CAD build for the part. Positions are in the model's coordinates, mm. Give positions to 0.01 mm unless a question says otherwise; leave off trailing zeros. Write each loop counter-clockwise with the first axis right and the second up, starting at its lowest first coordinate (ties: lowest second). Pieces come first, ordered by that corner, then holes. Notation, with made-up numbers: (-9.75, 60) - (44.25, 60) arc R18 ccw to (44.25, 75) - close; hole circle Ø6 at (3, 1.25). An arc over 180 degrees is marked (long way). Answer as a JSON object with one key per item and string values.
Autodesk Inventor part; units mm, degrees
ref_plane "YZ Plane" through (0, 0, 0) normal (1, 0, 0) x (0, 1, 0)
ref_plane "XZ Plane" through (0, 0, 0) normal (0, 1, 0) x (-1, 0, 0)
ref_plane "XY Plane" through (0, 0, 0) normal (0, 0, 1) x (1, 0, 0)
sketch "Esquisse1" plane through (0, 0, 0) normal (0, 1, 0) x (-1, 0, 0)
  line L0 (100, 500) -> (-100, 500)
  line L1 (-100, 500) -> (-100, -500)
  line L2 (-100, -500) -> (100, -500)
  line L3 (100, -500) -> (100, 500)
  point P0 (0, 0)
  dimension "d0" = 1000
  dimension "d1" = 200
  dimension "d4" = 500
  dimension "d5" = 100
extrude "Extrusion1" add sketch "Esquisse1" along normal blind 10
sketch "Esquisse2" plane through (0, 10, 0) normal (0, 1, 0) x (1, 0, 0)
  line L0 (100, -500) -> (100, 500)
  line L1 (100, -340) -> (40, -300)
  line L2 (40, -300) -> (40, 300)
  line L3 (40, 300) -> (100, 340)
  line L4 (-100, 500) -> (-100, -500)
  point P0 (0, 0)
  dimension "d6" = 600
  dimension "d7" = 300
  dimension "d8" = 140
  dimension "d9" = 160
  dimension "d10" = 160
extrude "Extrusion2" cut sketch "Esquisse2" against normal through all
fillet "Congé1" radius 20 4 edges at (40, 5, 300) (100, 5, 340) (40, 5, -300) (100, 5, -340)
sketch "Esquisse3" plane through (0, 10, 0) normal (0, 1, 0) x (1, 0, 0)
  circle A0 centre (-60, -485) radius 1.5
  circle A1 centre (60, -485) radius 1.5
  circle A2 centre (-60, 485) radius 1.5
  circle A3 centre (60, 485) radius 1.5
  line L0 (-100, -500) -> (100, -500)
  line L1 (100, 500) -> (-100, 500)
  line L2 (-100, 500) -> (-100, -500)
  line L3 (100, -500) -> (100, -350.7037)
  line L4 (100, 350.7037) -> (100, 500)
  point P0 (0, 0)
  dimension "d14" = 3
  dimension "d15" = 3
  dimension "d16" = 3
  dimension "d17" = 3
  dimension "d18" = 15
  dimension "d19" = 15
  dimension "d20" = 15
  dimension "d21" = 15
  dimension "d22" = 40
  dimension "d23" = 40
  dimension "d24" = 40
  dimension "d25" = 40
extrude "Extrusion3" cut sketch "Esquisse3" against normal through all
equation "\"d10\" = d9"
equation "\"d15\" = d14"
equation "\"d16\" = d14"
equation "\"d17\" = d14"
equation "\"d19\" = d18"
equation "\"d20\" = d18"
equation "\"d21\" = d18"
equation "\"d23\" = d22"
equation "\"d24\" = d22"
equation "\"d25\" = d22"
properties part number "Coté long plateau" material "Bois (bouleau)"
Item 1: Mould opens along Y. For faces 1 (the flat face through (-21, 10, 7)), 2 (the flat face through (-21, 0, 7)), 3 (the flat face through (70, 5, -320)) say: +Y half, -Y half, draft (parallel to the pull), parting line (faces both ways), or undercut.
Entries:
{"face 1": "+Y half", "face 2": "-Y half", "face 3": "draft"}
Item 2: Cut at B-B (z = -20). Give the cut face in (x, y).
Entries:
{"outline": "(-100, 0) - (40, 0) - (40, 10) - (-100, 10) - close"}
Item 3: Probe line 1 (X direction, y = 8, z = -485); line 2 (Z direction, x = -61, y = 2.75); line 3 (Z direction, x = 60, y = 8.25). List the from-to ranges inside material, lowest first. Write a range as from..to.
Entries:
{"line 1": "-100..-61.5, -58.5..58.5, 61.5..100", "line 2": "-500..-486.12, -483.88..483.88, 486.12..500", "line 3": "-500..-486.5, -483.5..-313.33, 313.33..483.5, 486.5..500"}
Item 4: Flat gauge pins, fed straight in: P1, Ø8, axis at x = 47, z = 153.5, coming from the +Y side; P2, Ø3, axis at y = 3.5, z = -23, coming from the +X side. Where does each tip first touch, or does it go through?
Entries:
{"P1": "through", "P2": "x = 40"}
Item 5: Cut at A-A (y = 7.5). Give the cut face in (x, z).
Entries:
{"outline": "(-100, -500) - (100, -500) - (100, -350.7) arc R20 ccw to (91.09, -334.06) - (48.91, -305.94) arc R20 cw to (40, -289.3) - (40, 289.3) arc R20 cw to (48.91, 305.94) - (91.09, 334.06) arc R20 ccw to (100, 350.7) - (100, 500) - (-100, 500) - close; hole circle Ø3 at (-60, -485); hole circle Ø3 at (-60, 485); hole circle Ø3 at (60, -485); hole circle Ø3 at (60, 485)"}
